The drawing under review shows one solid part. Ordinate dimensions are in mm from its lowest x, y, z. Give positions to 0.01 mm unless a question says otherwise; leave off trailing zeros. Write each loop counter-clockwise with the first axis right and the second up, starting at its lowest first coordinate (ties: lowest second). Pieces come first, ordered by that corner, then holes.
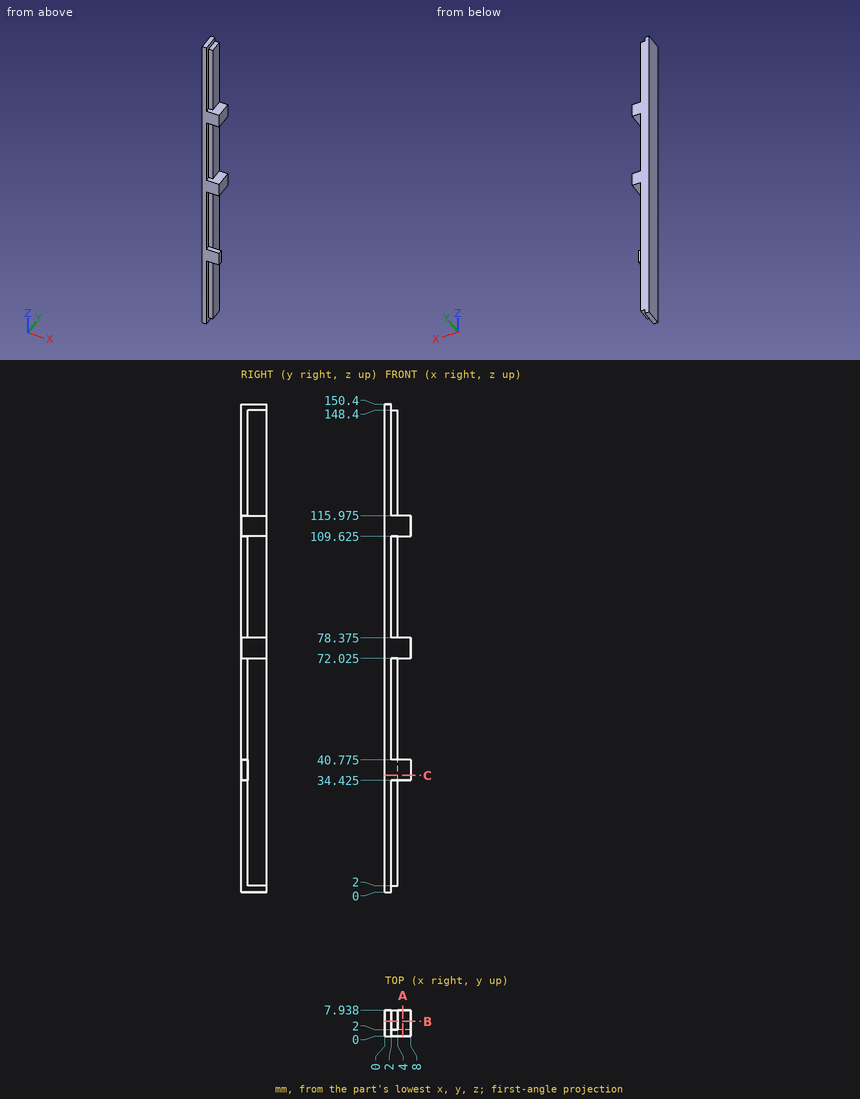
1) Consider section B-B, the plane y = 4.5. Give the boundary of the cut face in (x, z) (1 decimal).
2) Consider section C-C, the plane z = 36. Give the boundary of the cut face in (x, y).
3) Consider section A-A, the plane x = 5.5. Give the boundary of the cut face in (y, z) (1 decimal).
4) To check wall thickness, follow probe 1 along Z at (x, y) = (4, 1) (1 decimal); probe 2 along Z at (x, y) = (5, 4.5) (1 decimal); probe 3 along X at (y, z) = (2.5, 135.5). State the ranges of each line that lie inside material, in increasing order.
5) Insertion check: pin 1 (2 mm diameter, centred on x = 3.5, z = 136, fed in from -Y); pin 2 (1.8 mm diameter, centred on x = 5, y = 6, fed in from -Z) (1 decimal); pin 3 (2 mm diameter, centred on x = 5.5, z = 36.5, fed in from +Y); pin 4 (3 mm diameter, centred on x = 7, z = 80, fed in from +Y). Each pin has a flat end and moves straight along its axis. Give the tip position at first contact, or say it passes through.
Answer block:
1. outline: (0, 0) - (2, 0) - (2, 2) - (4, 2) - (4, 72) - (8, 72) - (8, 78.4) - (4, 78.4) - (4, 109.6) - (8, 109.6) - (8, 116) - (4, 116) - (4, 148.4) - (2, 148.4) - (2, 150.4) - (0, 150.4) - close
2. outline: (0, 0) - (8, 0) - (8, 2) - (4, 2) - (4, 7.94) - (0, 7.94) - close
3. outline: (0, 34.4) - (2, 34.4) - (2, 40.8) - (0, 40.8) - close; (0, 72) - (7.9, 72) - (7.9, 78.4) - (0, 78.4) - close; (0, 109.6) - (7.9, 109.6) - (7.9, 116) - (0, 116) - close
4. probe 1: z = 34.4 to 40.8, 72 to 78.4, 109.6 to 116
4. probe 2: z = 72 to 78.4, 109.6 to 116
4. probe 3: x = 0 to 4
5. pin 1: stops at y = 2
5. pin 2: stops at z = 72
5. pin 3: stops at y = 2
5. pin 4: passes through
